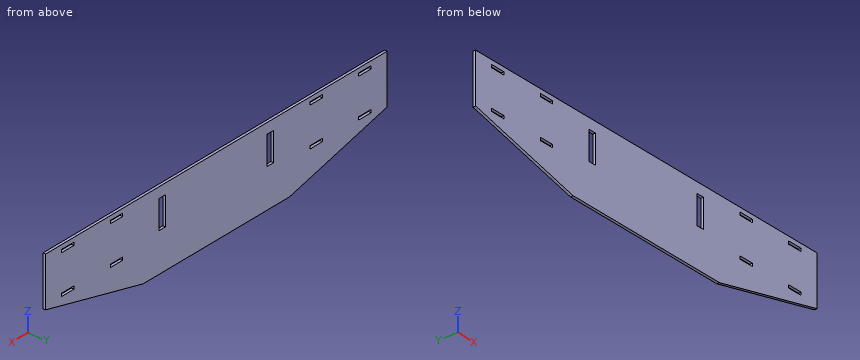
from build123d import *

# Parameters (mm, degrees)
SKETCH1_W           = 711.2
SKETCH1_H           = 139.7
BOSS_EXTRUDE1_DEPTH = 4.7625
CUT_EXTRUDE1_DEPTH  = 5.7625
SKETCH3_W           = 13.208
SKETCH3_H           = 51.308
CUT_EXTRUDE2_DEPTH  = 5.7625
SKETCH4_W           = 25.908
SKETCH4_H           = 5.2705
CUT_EXTRUDE3_DEPTH  = 5.7625


with BuildPart() as part:
    # Sketch1 → Boss-Extrude1 (new body)
    with BuildSketch(Plane(origin=(0, 0, 0), x_dir=(1, 0, 0), z_dir=(0, 1, 0))):
        with Locations((0, 69.85)):
            Rectangle(SKETCH1_W, SKETCH1_H)
    extrude(amount=BOSS_EXTRUDE1_DEPTH)

    # Sketch2 → Cut-Extrude1 (cut, through all)
    with BuildSketch(Plane(origin=(0, 4.7625, 0), x_dir=(1, 0, 0), z_dir=(0, 1, 0))):
        Polygon((-355.6, 88.9), (-152.4, 139.7), (-355.6, 139.7), align=None)
        Polygon((355.6, 139.7), (152.4, 139.7), (355.6, 88.9), align=None)
    extrude(amount=-CUT_EXTRUDE1_DEPTH, mode=Mode.SUBTRACT)

    # Sketch3 → Cut-Extrude2 (cut, through all)
    with BuildSketch(Plane(origin=(0, 0, 0), x_dir=(-1, 0, 0), z_dir=(0, -1, 0))):
        with Locations((-112.7125, 44.45)):
            Rectangle(SKETCH3_W, SKETCH3_H)
        with Locations((112.7125, 44.45)):
            Rectangle(SKETCH3_W, SKETCH3_H)
    extrude(amount=-CUT_EXTRUDE2_DEPTH, mode=Mode.SUBTRACT)

    # Sketch4 → Cut-Extrude3 (cut, through all)
    with BuildSketch(Plane.XZ):
        with Locations((-207.9625, -10.31875)):
            Rectangle(SKETCH4_W, SKETCH4_H)
        with Locations((-207.9625, -80.16875)):
            Rectangle(SKETCH4_W, SKETCH4_H)
        with Locations((-309.5625, -80.16875)):
            Rectangle(SKETCH4_W, SKETCH4_H)
        with Locations((-309.5625, -10.31875)):
            Rectangle(SKETCH4_W, SKETCH4_H)
        with Locations((207.9625, -80.16875)):
            Rectangle(SKETCH4_W, SKETCH4_H)
        with Locations((309.5625, -80.16875)):
            Rectangle(SKETCH4_W, SKETCH4_H)
        with Locations((309.5625, -10.31875)):
            Rectangle(SKETCH4_W, SKETCH4_H)
        with Locations((207.9625, -10.31875)):
            Rectangle(SKETCH4_W, SKETCH4_H)
    extrude(amount=-CUT_EXTRUDE3_DEPTH, mode=Mode.SUBTRACT)


solid = part.part
The listing builds one solid part. Answer for the finished solid, in the listing's coordinates (mm). Coordinates: 2 decimals unless noted, no trailing zeros. Write each loop counter-clockwise with the first axis right and the second up, starting at its lowest first coordinate (ties: lowest second). Pieces come first, ordered by that corner, then holes. Notation, with made-up numbers: M 70.25,28 L 116.25,28 A18 cw 116.25,62 Z; hole C -28.75,86 d10. An arc over 180 degrees is marked long. Use one line per item in the form item = value.
Item 1: Find section D-D, the plane z = -102. Give the vertices of the cut face in (x, y), plus the area to 3 significant figures.
Model answer:
outline = M -303.2,0 L 303.2,0 L 303.2,4.76 L -303.2,4.76 Z
area = 2,890 mm2
Item 2: Find section C-C, the plane x = 279. Give the vertices of the cut face in (y, z), plus the area to 3 significant figures.
Model answer:
outline = M 0,-108.05 L 4.76,-108.05 L 4.76,0 L 0,0 Z
area = 515 mm2
Item 3: Find section B-B, the plane y = 2.55. Give the number of separate pieces and of enclosed holes in the cut face, plus the area to 3 significant figures.
Model answer:
separate_pieces = 1
enclosed_holes = 10
area = 86,600 mm2
Item 4: Find the intervals of material crossed by probe 1 along X at (y, z) = (1.7, -37); probe 2 along X at (y, z) = (3.45, -8.5); probe 3 along Z at (x, y) = (108, 2.6), in increasing order.
Model answer:
probe_1 = -355.6 to -119.32, -106.11 to 106.11, 119.32 to 355.6
probe_2 = -355.6 to -322.52, -296.61 to -220.92, -195.01 to 195.01, 220.92 to 296.61, 322.52 to 355.6
probe_3 = -139.7 to -70.1, -18.8 to 0
Item 5: Find section A-A, the plane z = -25. Give the vertices of the cut face in (x, y).
Model answer:
outline = M -355.6,0 L -119.32,0 L -119.32,4.76 L -355.6,4.76 Z; M -106.11,0 L 106.11,0 L 106.11,4.76 L -106.11,4.76 Z; M 119.32,0 L 355.6,0 L 355.6,4.76 L 119.32,4.76 Z
